Part model, mm, in its own coordinate system. Face numbers are marked on the shaded views. Give positions to 0.01 mm unless a question says otherwise; leave off trailing zeros. Answer as a JSON object with one key per item and string values.
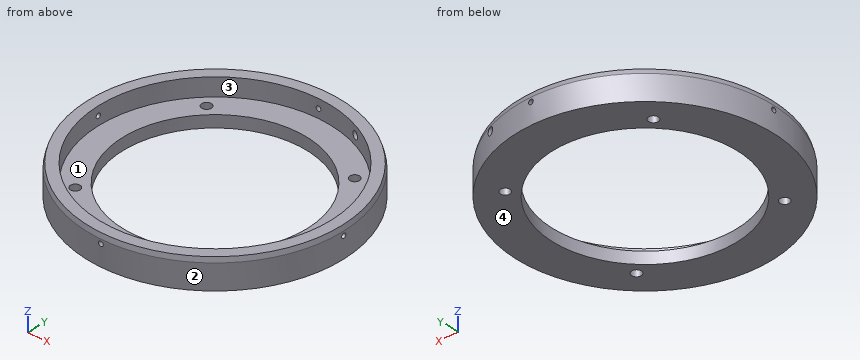
from build123d import *

# Parameters (mm, degrees)
SKETCH1_R                       = 68.1355
SKETCH1_R_2                     = 49.0855
EXTRUDE1_DEPTH                  = 15.875
SKETCH2_R                       = 61.7855
EXTRUDE2_DEPTH                  = 9.525
F_21_0_159_DIAMETER_HOLE1_D     = 4.0386
F_21_0_159_DIAMETER_HOLE1_DEPTH = 12.7
F_21_0_159_DIAMETER_HOLE1_TIP   = 1.213317848
CIRPATTERN1_COUNT               = 4
CIRPATTERN2_COUNT               = 4
CHAMFER1_SIZE                   = 2.54
CHAMFER1_SIZE2                  = 0.680590949


with BuildPart() as part:
    # Sketch1 → Extrude1 (new body)
    with BuildSketch(Plane.XY):
        Circle(SKETCH1_R)
        Circle(SKETCH1_R_2, mode=Mode.SUBTRACT)
    extrude(amount=EXTRUDE1_DEPTH)

    # Sketch2 → Extrude2 (cut)
    with BuildSketch(Plane.XY.offset(15.875)):
        Circle(SKETCH2_R)
    extrude(amount=-EXTRUDE2_DEPTH, mode=Mode.SUBTRACT)

    # #21 (0.159) Diameter Hole1
    with Locations(Plane(origin=(26.074327006, 62.948993887, 11.1125), x_dir=(-0.9238795325112864, 0.38268343236509067, 0), z_dir=(0.38268343236509067, 0.9238795325112864, 0))):
        with Locations((0, 0)):
            Hole(F_21_0_159_DIAMETER_HOLE1_D / 2, depth=F_21_0_159_DIAMETER_HOLE1_DEPTH)
            with Locations((0, 0, -(F_21_0_159_DIAMETER_HOLE1_DEPTH + F_21_0_159_DIAMETER_HOLE1_TIP / 2))):  # 118° drill point
                Cone(0, F_21_0_159_DIAMETER_HOLE1_D / 2, F_21_0_159_DIAMETER_HOLE1_TIP, mode=Mode.SUBTRACT)

    # Sketch4 → #39 (0.0995) Diameter Hole2 (revolve, cut)
    with BuildSketch(Plane(origin=(0, 68.1355, 11.1125), x_dir=(0, 0, 1), z_dir=(1, 0, 0))):
        Polygon((0, 0), (0, 13.459277521), (1.26365, 12.7), (1.26365, 0), align=None)
    f_39_0_0995_diameter_hole2 = revolve(axis=Axis((0, 74.4855, 11.1125), (0, -1, 0)), mode=Mode.SUBTRACT)

    # CirPattern1: #39 (0.0995) Diameter Hole2 ×4 about axis
    cirpattern1_axis = Axis((0, 0, 15.875), (0, 0, -1))
    for i in range(1, CIRPATTERN1_COUNT):
        add(f_39_0_0995_diameter_hole2.rotate(cirpattern1_axis, i * 360 / CIRPATTERN1_COUNT), mode=Mode.SUBTRACT)

    # Sketch8 → #7 (0.201) Diameter Hole1 (revolve, cut)
    with BuildSketch(Plane(origin=(39.198817968, 39.198817968, 11.1125), x_dir=(0, -1, 0), z_dir=(1, 0, 0))):
        Polygon((0, 0), (0, 14.233816902), (2.5527, 12.7), (2.5527, 0), align=None)
    f_7_0_201_diameter_hole1 = revolve(axis=Axis((39.198817968, 39.198817968, 17.4625), (0, 0, -1)), mode=Mode.SUBTRACT)

    # CirPattern2: #7 (0.201) Diameter Hole1 ×4 about axis
    cirpattern2_axis = Axis((0, 0, 0), (0, 0, 1))
    for i in range(1, CIRPATTERN2_COUNT):
        add(f_7_0_201_diameter_hole1.rotate(cirpattern2_axis, i * 360 / CIRPATTERN2_COUNT), mode=Mode.SUBTRACT)

    # Chamfer1
    chamfer1_edges = [part.edges().sort_by_distance(p)[0] for p in [
        (-68.1355, 0, 15.875),
    ]]
    chamfer1_side = [part.faces().sort_by_distance(p)[0] for p in [
        (-68.1355, 0, 7.9375),
    ]]
    chamfer(chamfer1_edges, length=CHAMFER1_SIZE, length2=CHAMFER1_SIZE2, reference=chamfer1_side[0])


solid = part.part
1. Probe line 1 along X through (y, z) = (-37.5, 5.5); line 2 along Z through (x, y) = (-11.5, -51); line 3 along Y through (x, z) = (0, 12.5). List the from-to ranges inside material, lowest first.
Worked answers:
{"line 1": "x = -56.89 to -41.1, -37.29 to -31.67, 31.67 to 37.29, 41.1 to 56.89", "line 2": "z = 0 to 6.35", "line 3": "y = -68.14 to -61.79, 61.79 to 68.14"}
2. Two-plate mould, pull along X, no slides. Class the marked faces 1, 2, 3 and 4: +X half, -X half, draft (parallel to the pull), parting line (faces both ways), or undercut.
Worked answers:
{"face 1": "undercut", "face 2": "parting line", "face 3": "undercut", "face 4": "draft"}
3. Pin check, flat tips, straight feed: P1, Ø4, axis at x = 0, z = 11.11, coming from the -Y side; P2, Ø3, axis at x = -39.2, y = -39.2, coming from the -Z side; P3, Ø1.5, axis at x = -30, z = 11, coming from the +Y side; P4, Ø3, axis at x = -46.5, z = 10, coming from the +Y side. Stop position of each tip, or through.
Worked answers:
{"P1": "stops at y = -68.14", "P2": "passes through", "P3": "stops at y = 61.54", "P4": "stops at y = 51.16"}
